Here's how the part is built. I have some questions about the finished solid (model axes, mm). A direction names the side the tool comes from. Round coordinates to 2 decimals unless told otherwise and drop trailing zeros. Loops run counter-clockwise (first coordinate to the right, second up) from the corner with the lowest first, then second, coordinate; pieces in that order, holes last. Notation, with made-up numbers: (79.5, 87) -> (94.5, 87) arc R28 ccw to (94.5, 114) -> close; hole circle Ø4 at (41, 54). An arc over 180 degrees is marked (long way). Use one line per item in the form item = value. Start each with the question number.
Item 1: For faces 1 (the face through (-20, 7, 0)), 2 (the face through (1, 13, 0)), which set-ups out of +Z, -Z, +X, -X, +Y, -Y let a thin tool reach every point of the face, with its end or its side?
Item 2: If I drill on L1, parallel to Y at x = -15.5, z = 4.25, over which ranges is the centre line in solid material (lowest first)? Write a range as [from, to].
Item 3: If we section it at A-A (x = -2.5): Write out the boundary of the cut face in (y, z).
Item 4: Thinking about a two-plate mould opening in X: for faces 3 (the face through (20, 7, 0)), 4 (the face through (0, 7, -12.5)), 5 (the face through (-3, 13, 1)), which applies, released by +X, released by -X, zero draft, split by the parting line, or undercut?
Autodesk Inventor part; units mm, degrees
ref_plane "YZ Plane" through (0, 0, 0) normal (1, 0, 0) x (0, 1, 0)
ref_plane "XZ Plane" through (0, 0, 0) normal (0, 1, 0) x (-1, 0, 0)
ref_plane "XY Plane" through (0, 0, 0) normal (0, 0, 1) x (1, 0, 0)
sketch "Sketch1" plane through (0, 0, 0) normal (0, 1, 0) x (-1, 0, 0)
  line L0 (20, 12.5) -> (-20, 12.5)
  line L1 (-20, 12.5) -> (-20, -12.5)
  line L2 (-20, -12.5) -> (20, -12.5)
  line L3 (20, -12.5) -> (20, 12.5)
  line L4 (20, 12.5) -> (-20, -12.5) construction
  line L5 (-20, 12.5) -> (20, -12.5) construction
  point P0 (0, 0)
  dimension "d0" = 40
  dimension "d1" = 25
extrude "Extrusion1" add sketch "Sketch1" along normal blind 14
sketch "Sketch2" plane through (0, 14, 0) normal (0, 1, 0) x (1, 0, 0)
  line L0 (-18.5392, 5.6526) -> (18.5392, 5.6526) construction
  line L1 (18.5392, 5.6526) -> (18.5392, -5.6526) construction
  line L2 (18.5392, -5.6526) -> (-18.5392, -5.6526) construction
  line L3 (-18.5392, -5.6526) -> (-18.5392, 5.6526) construction
  line L4 (20, -12.5) -> (20, 12.5)
  line L5 (20, 12.5) -> (-20, 12.5)
  line L6 (-20, 12.5) -> (-20, -12.5)
  line L7 (-20, -12.5) -> (20, -12.5)
  spline S0 degree 2 poles (-9.6413, 0.5796) (-9.6413, -0.7899) (-10.7516, -2.9941) (-11.6835, -3.61) knots 0 0 0 1 2 2 2
  spline S1 degree 2 poles (-11.6835, -3.61) (-12.4452, -4.0881) (-14.0093, -4.4123) (-15.2248, -4.4123) knots 0 0 0 1 2 2 2
  line L8 (-15.2248, -4.4123) -> (-17.5263, -4.4123)
  line L9 (-17.5263, -4.4123) -> (-17.5263, 5.5877)
  line L10 (-17.5263, 5.5877) -> (-15.2491, 5.5877)
  spline S2 degree 2 poles (-15.2491, 5.5877) (-13.8391, 5.5877) (-12.2345, 5.1663) (-11.6673, 4.7936) knots 0 0 0 1 2 2 2
  spline S3 degree 2 poles (-11.6673, 4.7936) (-10.7029, 4.1534) (-9.6413, 2.0383) (-9.6413, 0.5796) knots 0 0 0 1 2 2 2
  spline S4 degree 2 poles (-11.0271, 0.5958) (-11.0271, 1.7466) (-11.7888, 3.3754) (-12.5425, 3.8373) knots 0 0 0 1 2 2 2
  spline S5 degree 2 poles (-12.5425, 3.8373) (-13.0773, 4.1534) (-14.2848, 4.437) (-15.1843, 4.437) knots 0 0 0 1 2 2 2
  line L11 (-15.1843, 4.437) -> (-16.1973, 4.437)
  line L12 (-16.1973, 4.437) -> (-16.1973, -3.2615)
  line L13 (-16.1973, -3.2615) -> (-15.1843, -3.2615)
  spline S6 degree 2 poles (-15.1843, -3.2615) (-14.301, -3.2615) (-12.9639, -2.9779) (-12.4209, -2.597) knots 0 0 0 1 2 2 2
  spline S7 degree 2 poles (-12.4209, -2.597) (-11.724, -2.127) (-11.0271, -0.5711) (-11.0271, 0.5958) knots 0 0 0 1 2 2 2
  line L14 (-4.3172, 1.7385) -> (-4.382, 1.7385)
  spline S8 degree 2 poles (-4.382, 1.7385) (-4.5279, 1.779) (-4.8439, 1.7952) (-5.0627, 1.7952) knots 0 0 0 1 2 2 2
  spline S9 degree 2 poles (-5.0627, 1.7952) (-5.5733, 1.7952) (-6.5781, 1.3495) (-7.0319, 0.9119) knots 0 0 0 1 2 2 2
  line L15 (-7.0319, 0.9119) -> (-7.0319, -4.4123)
  line L16 (-7.0319, -4.4123) -> (-8.2961, -4.4123)
  line L17 (-8.2961, -4.4123) -> (-8.2961, 3.0918)
  line L18 (-8.2961, 3.0918) -> (-7.0319, 3.0918)
  line L19 (-7.0319, 3.0918) -> (-7.0319, 1.9735)
  spline S10 degree 2 poles (-7.0319, 1.9735) (-6.3431, 2.5894) (-5.314, 3.0918) (-4.8277, 3.0918) knots 0 0 0 1 2 2 2
  spline S11 degree 2 poles (-4.8277, 3.0918) (-4.6332, 3.0918) (-4.4387, 3.0756) (-4.3172, 3.0513) knots 0 0 0 1 2 2 2
  line L20 (-4.3172, 3.0513) -> (-4.3172, 1.7385)
  line L21 (-2.0481, -4.4123) -> (-3.3123, -4.4123)
  line L22 (-3.3123, -4.4123) -> (-3.3123, 3.0918)
  line L23 (-3.3123, 3.0918) -> (-2.0481, 3.0918)
  line L24 (-2.0481, 3.0918) -> (-2.0481, -4.4123)
  line L25 (-1.959, 4.3398) -> (-3.3934, 4.3398)
  line L26 (-3.3934, 4.3398) -> (-3.3934, 5.6526)
  line L27 (-3.3934, 5.6526) -> (-1.959, 5.6526)
  line L28 (-1.959, 5.6526) -> (-1.959, 4.3398)
  line L29 (5.699, 3.0918) -> (2.8708, -4.4123)
  line L30 (2.8708, -4.4123) -> (1.7363, -4.4123)
  line L31 (1.7363, -4.4123) -> (-1.0676, 3.0918)
  line L32 (-1.0676, 3.0918) -> (0.3019, 3.0918)
  line L33 (0.3019, 3.0918) -> (2.3522, -2.6862)
  line L34 (2.3522, -2.6862) -> (4.3862, 3.0918)
  line L35 (4.3862, 3.0918) -> (5.699, 3.0918)
  spline S12 degree 2 poles (9.913, -4.5824) (8.1139, -4.5824) (6.1366, -2.5646) (6.1366, -0.7008) knots 0 0 0 1 2 2 2
  spline S13 degree 2 poles (6.1366, -0.7008) (6.1366, 1.1307) (8.0572, 3.3025) (9.605, 3.3025) knots 0 0 0 1 2 2 2
  spline S14 degree 2 poles (9.605, 3.3025) (10.3019, 3.3025) (11.3797, 2.8973) (11.7768, 2.4678) knots 0 0 0 1 2 2 2
  spline S15 degree 2 poles (11.7768, 2.4678) (12.182, 2.0383) (12.6115, 0.7984) (12.6115, -0.1011) knots 0 0 0 1 2 2 2
  line L36 (12.6115, -0.1011) -> (12.6115, -0.7899)
  line L37 (12.6115, -0.7899) -> (7.417, -0.7899)
  spline S16 degree 2 poles (7.417, -0.7899) (7.417, -2.0946) (8.7298, -3.4803) (9.8967, -3.4803) knots 0 0 0 1 2 2 2
  spline S17 degree 2 poles (9.8967, -3.4803) (10.31, -3.4803) (11.1123, -3.294) (11.4365, -3.1481) knots 0 0 0 1 2 2 2
  spline S18 degree 2 poles (11.4365, -3.1481) (11.7768, -2.986) (12.2468, -2.7024) (12.4008, -2.5727) knots 0 0 0 1 2 2 2
  line L38 (12.4008, -2.5727) -> (12.4737, -2.5727)
  line L39 (12.4737, -2.5727) -> (12.4737, -3.9504)
  spline S19 degree 2 poles (12.4737, -3.9504) (12.2549, -4.0395) (11.5904, -4.2988) (11.3311, -4.3717) knots 0 0 0 1 2 2 2
  spline S20 degree 2 poles (11.3311, -4.3717) (10.9664, -4.4771) (10.3668, -4.5824) (9.913, -4.5824) knots 0 0 0 1 2 2 2
  spline S21 degree 2 poles (11.3797, 0.1744) (11.3635, 0.685) (11.1528, 1.4305) (10.9502, 1.6817) knots 0 0 0 1 2 2 2
  spline S22 degree 2 poles (10.9502, 1.6817) (10.7314, 1.9654) (10.0426, 2.2652) (9.5321, 2.2652) knots 0 0 0 1 2 2 2
  spline S23 degree 2 poles (9.5321, 2.2652) (9.0296, 2.2652) (8.3246, 1.9654) (8.0329, 1.6736) knots 0 0 0 1 2 2 2
  spline S24 degree 2 poles (8.0329, 1.6736) (7.7493, 1.3738) (7.4575, 0.6526) (7.417, 0.1744) knots 0 0 0 1 2 2 2
  line L40 (7.417, 0.1744) -> (11.3797, 0.1744)
  line L41 (17.8708, 1.7385) -> (17.806, 1.7385)
  spline S25 degree 2 poles (17.806, 1.7385) (17.6601, 1.779) (17.3441, 1.7952) (17.1253, 1.7952) knots 0 0 0 1 2 2 2
  spline S26 degree 2 poles (17.1253, 1.7952) (16.6147, 1.7952) (15.6099, 1.3495) (15.1561, 0.9119) knots 0 0 0 1 2 2 2
  line L42 (15.1561, 0.9119) -> (15.1561, -4.4123)
  line L43 (15.1561, -4.4123) -> (13.8919, -4.4123)
  line L44 (13.8919, -4.4123) -> (13.8919, 3.0918)
  line L45 (13.8919, 3.0918) -> (15.1561, 3.0918)
  line L46 (15.1561, 3.0918) -> (15.1561, 1.9735)
  spline S27 degree 2 poles (15.1561, 1.9735) (15.8449, 2.5894) (16.8741, 3.0918) (17.3603, 3.0918) knots 0 0 0 1 2 2 2
  spline S28 degree 2 poles (17.3603, 3.0918) (17.5548, 3.0918) (17.7493, 3.0756) (17.8708, 3.0513) knots 0 0 0 1 2 2 2
  line L47 (17.8708, 3.0513) -> (17.8708, 1.7385)
  point P0 (0, 0)
  point P1 (-18.5392, 0)
  point P2 (-20, 0)
  point P3 (0, 5.6526)
  point P4 (0, 12.5)
extrude "Extrusion2" cut sketch "Sketch2" against normal blind 1 contours S0 S1 L8 L9 L10 S2 S3 | L14 S8 S9 L15 L16 L17 L18 L19 S10 S11 L20 | L21 L22 L23 L24 | L25 L26 L27 L28 | L29 L30 L31 L32 L33 L34 L35 | S12 S13 S14 S15 L36 L37 S16 S17 S18 L38 L39 S19 S20 | L41 S25 S26 L42 L43 L44 L45 L46 S27 S28 L47
properties part number "Motor Driver"
Values found:
q1.face_1 = +Z, -Z, -X, +Y, -Y
q1.face_2 = +Y
q2.L1 = [0, 13]
q3.outline = (0, -12.5) -> (14, -12.5) -> (14, -5.65) -> (13, -5.65) -> (13, -4.34) -> (14, -4.34) -> (14, -3.09) -> (13, -3.09) -> (13, 4.41) -> (14, 4.41) -> (14, 12.5) -> (0, 12.5) -> close
q4.face_3 = released by +X
q4.face_4 = zero draft
q4.face_5 = undercut
